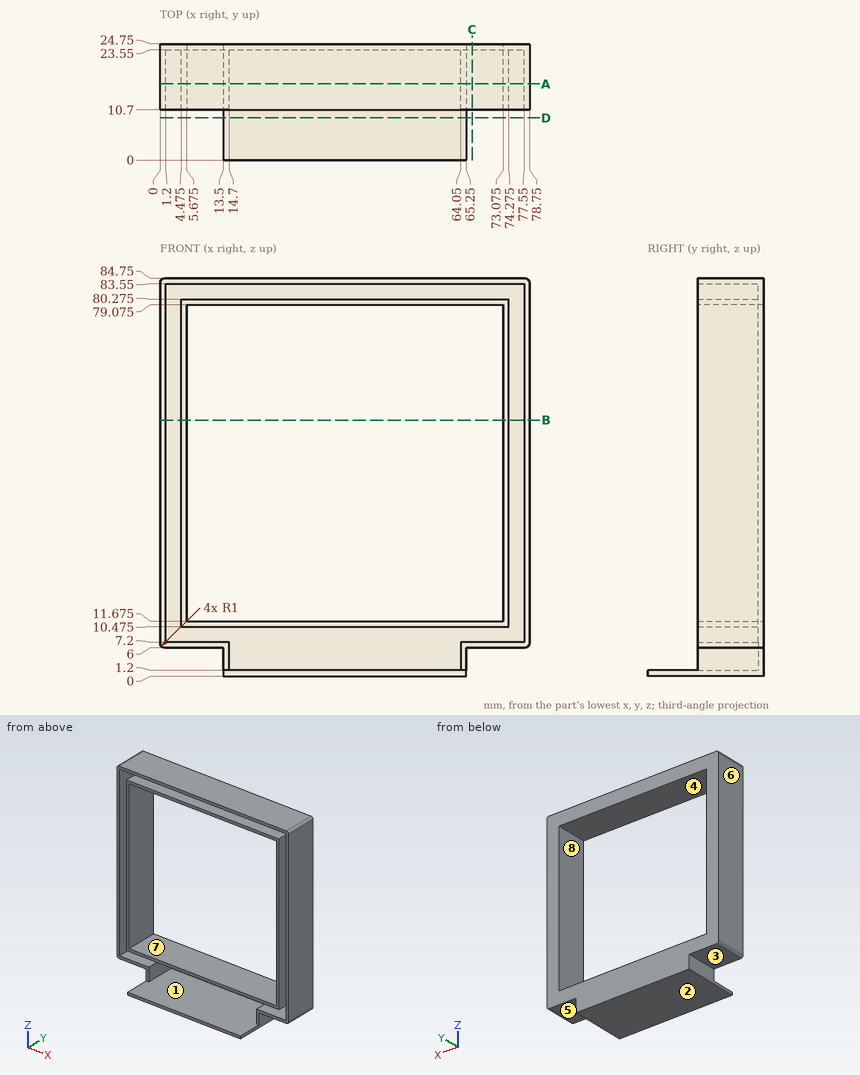
Here's the drawing with two shaded views (mm, measured from the low corner). I have some questions. A direction names the side the tool comes from. Give positions to 0.01 mm unless a question says otherwise; leave off trailing zeros. Write each loop counter-clockwise with the first axis right and the second up, starting at its lowest first coordinate (ties: lowest second). Pieces come first, ordered by that corner, then holes. Notation, with made-up numbers: (86, -37.75) - (110, -37.75) arc R26 ccw to (110, -9.75) - close; hole circle Ø5 at (84, -18.75). An arc over 180 degrees is marked (long way). Write item = value, one per line. Start each with the question number.
1. Imagine slicing it at B-B (z = 54.5). Please give me the cut outline in (x, y) (3 decimals).
2. On a 3-axis mill with a long thin cutter (end or side, diameter ignored), from which of +Z, -Z, +X, -X, +Y, -Y can I reach the whole of each face in a straight line? I mean the marked faces 1, 2, 3 and 4. Say none if no direction works.
3. Thinking about a two-plate mould opening in Z: for the marked faces 5, 6, 7 and 8, which applies, released by +Z, released by -Z, zero draft, split by the parting line, or undercut?
4. Imagine slicing it at C-C (x = 66.5). Please give me the cut outline in (y, z) (3 decimals).
5. Imagine slicing it at A-A (y = 16.25). Please give me the cut outline in (x, z) (3 decimals), and give its area (3 significant figures).
6. Imagine slicing it at D-D (y = 9). Please give me the cut outline in (x, z), and give its area (3 significant figures).
7. Please list where these lines run through material, in increasing order: line 1 (Z direction, x = 27, y = 18) (3 decimals); line 2 (X direction, y = 21, z = 69) (3 decimals); line 3 (Z direction, x = 71, y = 13.75) (3 decimals).
8. For pin 1 (1 mm diameter, centred on x = 66.5, y = 14, fed in from -Z); pin 2 (1.8 mm diameter, centred on y = 14, z = 2, fed in from +X); pin 3 (1.8 mm diameter, centred on y = 13.5, z = 3.5, fed in from -X); pin 4 (23 mm diameter, centred on x = 41.5, z = 32, fed in from -Y), each with a flat end and sliding along its axis, tell me the tip position at first contact or that it passes through.
Worked answers:
q1.outline = (0, 10.7) - (1.2, 10.7) - (1.2, 23.55) - (4.475, 23.55) - (4.475, 10.7) - (5.675, 10.7) - (5.675, 24.75) - (0, 24.75) - close; (73.075, 10.7) - (74.275, 10.7) - (74.275, 23.55) - (77.55, 23.55) - (77.55, 10.7) - (78.75, 10.7) - (78.75, 24.75) - (73.075, 24.75) - close
q2.face_1 = -Y
q2.face_2 = -Z, +X, -X, +Y, -Y
q2.face_3 = -Z, -X, +Y, -Y
q2.face_4 = +Y, -Y
q3.face_5 = released by -Z
q3.face_6 = zero draft
q3.face_7 = undercut
q3.face_8 = undercut
q4.outline = (10.7, 6) - (24.75, 6) - (24.75, 11.675) - (10.7, 11.675) - (10.7, 10.475) - (23.55, 10.475) - (23.55, 7.2) - (10.7, 7.2) - close; (10.7, 79.075) - (24.75, 79.075) - (24.75, 84.75) - (10.7, 84.75) - (10.7, 83.55) - (23.55, 83.55) - (23.55, 80.275) - (10.7, 80.275) - close
q5.outline = (0, 7) arc R1 ccw to (1, 6) - (13.5, 6) - (13.5, 0) - (65.25, 0) - (65.25, 6) - (77.75, 6) arc R1 ccw to (78.75, 7) - (78.75, 83.75) arc R1 ccw to (77.75, 84.75) - (1, 84.75) arc R1 ccw to (0, 83.75) - close; (4.475, 10.475) - (74.275, 10.475) - (74.275, 80.275) - (4.475, 80.275) - close; hole (1.2, 7.2) - (14.7, 7.2) - (14.7, 1.2) - (64.05, 1.2) - (64.05, 7.2) - (77.55, 7.2) - (77.55, 83.55) - (1.2, 83.55) - close; hole (5.675, 11.675) - (73.075, 11.675) - (73.075, 79.075) - (5.675, 79.075) - close
q5.area = 715 mm2
q6.outline = (13.5, 0) - (65.25, 0) - (65.25, 1.2) - (13.5, 1.2) - close
q6.area = 62.1 mm2
q7.line_1 = 0 to 1.2, 10.475 to 11.675, 79.075 to 80.275, 83.55 to 84.75
q7.line_2 = 0 to 1.2, 4.475 to 5.675, 73.075 to 74.275, 77.55 to 78.75
q7.line_3 = 6 to 7.2, 10.475 to 11.675, 79.075 to 80.275, 83.55 to 84.75
q8.pin_1 = 6
q8.pin_2 = 65.25
q8.pin_3 = 13.5
q8.pin_4 = through
